from build123d import *

# Parameters (mm, degrees)
F0_W          = 100
F0_H          = 100
F1_DEPTH      = 50
F4_DEPTH      = 50
F5_W          = 13
F5_H          = 50
F6_DEPTH      = 30
F8_R          = 10.8467438632
F9_DEPTH      = 35
F10_T4_DEPTH  = 268.9949493661
F10_T9_DEPTH  = 268.9949493661
F10_T14_DEPTH = 268.9949493661
F10_T20_DEPTH = 268.9949493661


# Not quite as in the source:
# - a fillet or chamfer that OpenCascade refuses, or shapes differently, is made with other operations: its cross-section is extruded or revolved along the edge and cut away or added


with BuildPart() as f1:
    # F0 (on Top) → F1 (new body)
    with BuildSketch(Plane.XY):
        Rectangle(F0_W, F0_H)
    extrude(amount=F1_DEPTH)

    # F3 (on offset) → F4 (join)
    with BuildSketch(Plane.XY.offset(50)):
        Polygon((49.7613176703, 49.4384859949), (-50.2386823297, 49.4384859949), (-50.2386823297, 27.4384859949), (-42.6304154098, 27.4384859949), (49.7613176703, 27.4384859949), align=None)
    extrude(amount=F4_DEPTH)

    # F5 (on offset) → F6 (join)
    with BuildSketch(Plane.XY.offset(50)):
        with Locations((-42.9296287298, 0.3518681973)):
            Rectangle(F5_W, F5_H)
    extrude(amount=F6_DEPTH)

    # F7: F1 across plane


with BuildPart() as f1_1:
    add(f1.part)
    add(f1.part.mirror(Plane.YZ))

    # F8 (on Right) → F9 (join, symmetric)
    with BuildSketch(Plane.YZ):
        with Locations((23.399380967, 57.991553098)):
            Circle(F8_R)
    extrude(amount=F9_DEPTH, both=True)

    # F10: fillet of radius 33.7989898732 on 1 edges, made by hand


with BuildPart() as f10_tool2:
    # F10_s3 → F10_t4 (new body)
    with BuildSketch(Plane.YZ.offset(-134.4974746831)):
        with BuildLine():
            ThreePointArc((-50, 16.2010101268), (-40.1005050634, 40.1005050634), (-16.2010101268, 50))
            Line((-16.2010101268, 50), (-50, 50))
            Line((-50, 50), (-50, 16.2010101268))
        make_face()
    extrude(amount=F10_T4_DEPTH)

    split(bisect_by=Plane.XZ.offset(24.6481318027), keep=Keep.TOP)


with BuildPart() as f1_2:
    add(f1_1.part)

    # F10_t1: cut F10_tool2
    add(f10_tool2.part, mode=Mode.SUBTRACT)


with BuildPart() as f10_tool7:
    # F10_s8 → F10_t9 (new body)
    with BuildSketch(Plane.YZ.offset(-134.4974746831)):
        with BuildLine():
            ThreePointArc((-50, 16.2010101268), (-40.1005050634, 40.1005050634), (-16.2010101268, 50))
            Line((-16.2010101268, 50), (-50, 50))
            Line((-50, 50), (-50, 16.2010101268))
        make_face()
    extrude(amount=F10_T9_DEPTH)

    split(bisect_by=Plane.YZ.offset(-49.4296287298), keep=Keep.BOTTOM)


with BuildPart() as f1_3:
    add(f1_2.part)

    # F10_t6: cut F10_tool7
    add(f10_tool7.part, mode=Mode.SUBTRACT)


with BuildPart() as f10_tool12:
    # F10_s13 → F10_t14 (new body)
    with BuildSketch(Plane.YZ.offset(-134.4974746831)):
        with BuildLine():
            ThreePointArc((-50, 16.2010101268), (-40.1005050634, 40.1005050634), (-16.2010101268, 50))
            Line((-16.2010101268, 50), (-50, 50))
            Line((-50, 50), (-50, 16.2010101268))
        make_face()
    extrude(amount=F10_T14_DEPTH)

    split(bisect_by=Plane.YZ.offset(-36.4296287298), keep=Keep.TOP)

    split(bisect_by=Plane.YZ.offset(36.4296287298), keep=Keep.BOTTOM)


with BuildPart() as f1_4:
    add(f1_3.part)

    # F10_t11: cut F10_tool12
    add(f10_tool12.part, mode=Mode.SUBTRACT)


with BuildPart() as f10_tool18:
    # F10_s19 → F10_t20 (new body)
    with BuildSketch(Plane.YZ.offset(-134.4974746831)):
        with BuildLine():
            ThreePointArc((-50, 16.2010101268), (-40.1005050634, 40.1005050634), (-16.2010101268, 50))
            Line((-16.2010101268, 50), (-50, 50))
            Line((-50, 50), (-50, 16.2010101268))
        make_face()
    extrude(amount=F10_T20_DEPTH)

    split(bisect_by=Plane.YZ.offset(49.4296287298), keep=Keep.TOP)


with BuildPart() as f1_5:
    add(f1_4.part)

    # F10_t17: cut F10_tool18
    add(f10_tool18.part, mode=Mode.SUBTRACT)


solid = f1_5.part
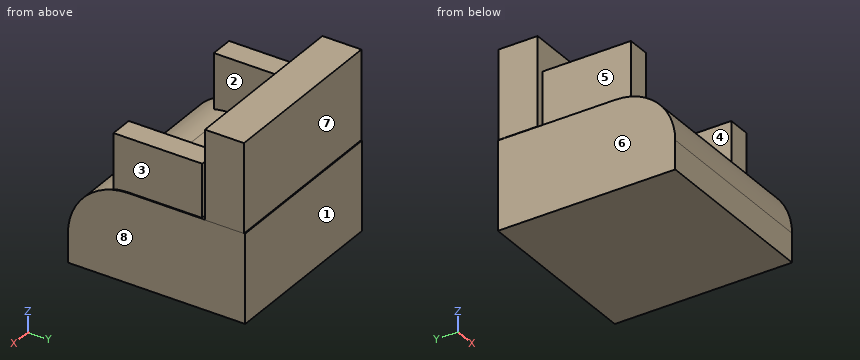
The listing builds one solid part. Answer for the finished solid, in the listing's coordinates (mm). Face numbers are marked on the shaded views. A direction names the side the tool comes from. Give positions to 0.01 mm unless a question says otherwise; leave off trailing zeros. Loops run counter-clockwise (first coordinate to the right, second up) from the corner with the lowest first, then second, coordinate; pieces in that order, holes last. Notation, with made-up numbers: M 74.25,-25.5 L 79.25,-25.5 A27 ccw 79.25,9.5 Z; hole C -28,-33.5 d6. An arc over 180 degrees is marked long. Answer as CSV lines item,"result".
Item 1: Straight lines are drawn through the part: line 1 along X through (y, z) = (13, 76.5); line 2 along Z through (x, y) = (26, 1); line 3 along Z through (x, y) = (45, -13). For each, find the intervals that lie inside material, in ascending order. Write a range as [from, to].
Values follow:
line 1,"x = [-49.43, -36.43], [36.43, 49.43]"
line 2,"z = [0, 50]"
line 3,"z = [0, 80]"
Item 2: Which of the six approach directions +Z, -Z, +X, -X, +Y, -Y give full straight-line access (tool end or side, diameter ignored) to the marked faces 5, 6, 7 and 8?
Values follow:
face 5,"+Z, -X, -Y"
face 6,"-Z, -X, +Y, -Y"
face 7,"+Z, +X, -X, +Y"
face 8,"-Z, +X, +Y, -Y"
Item 3: The part is cut by section C-C (y = -8.5). Give the vertices of the cut face in (x, z), and give its area (3 significant figures).
Values follow:
outline,"M -50,0 L 50,0 L 50,50 L 49.43,50 L 49.43,80 L 36.43,80 L 36.43,50 L -36.43,50 L -36.43,80 L -49.43,80 L -49.43,50 L -50,50 Z"
area,"5,780 mm^2"
Item 4: The mould has two halves that part along X. Classify the marked faces 1, 2, 3 and 4: released by +X, released by -X, zero draft, split by the parting line, or undercut.
Values follow:
face 1,"zero draft"
face 2,"undercut"
face 3,"released by +X"
face 4,"undercut"
Item 5: The part is cut by section A-A (z = 64.5). Give the vertices of the cut face in (x, y).
Values follow:
outline,"M -50.24,27.44 L -35,27.44 L -35,14.72 L 35,14.72 L 35,27.44 L 50.24,27.44 L 50.24,49.44 L -50.24,49.44 Z; M -49.43,-24.65 L -36.43,-24.65 L -36.43,25.35 L -49.43,25.35 Z; M 36.43,-24.65 L 49.43,-24.65 L 49.43,25.35 L 36.43,25.35 Z"
Item 6: Given pin 1 Ø10 at (y, z) = (6.5, 64.5) entering from -X; pin 2 Ø1.5 at (y, z) = (7, 21.5) entering from -X; pin 3 Ø10.5 at (x, y) = (40.5, -9) entering from +Z, each flat-ended and moving along its own axis, determine where each tip first touches the part or whether it passes through.
Values follow:
pin 1,"stops at x = -49.43"
pin 2,"stops at x = -50"
pin 3,"stops at z = 80"
Item 7: The part is cut by section B-B (x = 42). Give the vertices of the cut face in (y, z), and give its area (3 significant figures).
Values follow:
outline,"M -50,0 L 50,0 L 50,50 L 49.44,50 L 49.44,100 L 27.44,100 L 27.44,50 L 25.35,50 L 25.35,80 L -24.65,80 L -24.65,48.93 A33.8 ccw -50,16.2 Z"
area,"7,360 mm^2"
Item 8: The part is cut by section D-D (z = 91). Give the vertices of the cut face in (x, y), and give its area (3 significant figures).
Values follow:
outline,"M -50.24,27.44 L 50.24,27.44 L 50.24,49.44 L -50.24,49.44 Z"
area,"2,210 mm^2"
